Input: part model. Units: mm. Frame: model coordinates. A direction names the side the tool comes from. Give positions to 0.01 mm unless a question says otherwise; leave off trailing zeros. Loops run counter-clockwise (first coordinate to the right, second up) from the corner with the lowest first, then second, coordinate; pieces in that order, holes last. Notation, with made-up numbers: M 0.5,66 L 46.5,66 A6 ccw 46.5,76 Z; hole C 50,76.5 d8. An arc over 180 degrees is marked long. Return JSON: item names as keys, results as strings. Group by question number.
```python
from build123d import *

# Parameters (mm, degrees)
PAD002_DEPTH     = 75
BOX011_W         = 66
BOX011_H         = 16
BOX011_DEPTH     = 0.75
BOX010_W         = 0.75
BOX010_H         = 0.75
BOX010_DEPTH     = 9
ARRAY007_X_COUNT = 2
ARRAY007_X_PITCH = 70.45
ARRAY007_Y_COUNT = 2
ARRAY007_Y_PITCH = 24.45
BOX009_W         = 71.2
BOX009_H         = 25.2
BOX009_DEPTH     = 8.9


with BuildPart() as screen_lateral_hole:
    # Sketch002 → Pad002 (new body)
    with BuildSketch(Plane.YZ):
        Polygon((12.982779, 1.619702), (12.982779, 4.769702), (15.482779, 4.769702), (15.482779, 6.269702), (30.482779, 6.269702), (30.482779, 4.769702), (32.982779, 4.769702), (32.982779, 1.619702), align=None)
    extrude(amount=PAD002_DEPTH)


with BuildPart() as screen_lateral_hole_1:
    # Body002 placement: moved
    add(screen_lateral_hole.part.moved(Location((9, 0, 0))))


with BuildPart() as screen:
    # Box011 → Box011 (new body)
    with BuildSketch(Plane(origin=(9, 15, 9.75), x_dir=(1, 0, 0), z_dir=(0, 0, 1))):
        with Locations((33, 8)):
            Rectangle(BOX011_W, BOX011_H)
    extrude(amount=BOX011_DEPTH)


with BuildPart() as obj1:
    # Box010 → Box010 (new body)
    with BuildSketch(Plane(origin=(6.4, 10.4, 1.6), x_dir=(1, 0, 0), z_dir=(0, 0, 1))):
        with Locations((0.375, 0.375)):
            Rectangle(BOX010_W, BOX010_H)
    extrude(amount=BOX010_DEPTH)

    # Array007 X: obj1_2


with BuildPart() as obj1_1:
    add(obj1.part)
    with Locations(*[(i * ARRAY007_X_PITCH, 0, 0) for i in range(1, ARRAY007_X_COUNT)]):
        add(obj1.part)

    # Array007 Y: obj1_2


with BuildPart() as obj1_2:
    add(obj1_1.part)
    with Locations(*[(0, i * ARRAY007_Y_PITCH, 0) for i in range(1, ARRAY007_Y_COUNT)]):
        add(obj1_1.part)

    # Fusion002004: union Screen Lateral Hole, Screen
    add(screen_lateral_hole_1.part)
    add(screen.part)


with BuildPart() as panel:
    # Box009 → Box009 (new body)
    with BuildSketch(Plane(origin=(6.4, 10.4, 1.6), x_dir=(1, 0, 0), z_dir=(0, 0, 1))):
        with Locations((35.6, 12.6)):
            Rectangle(BOX009_W, BOX009_H)
    extrude(amount=BOX009_DEPTH)

    # Cut001: cut obj1
    add(obj1_2.part, mode=Mode.SUBTRACT)


solid = panel.part
```
Item 1: Section B-B, the plane z = 5.5. Return loops of the section in (x, y).
Item 2: Section A-A, the plane x = 51.5. Return loops of the section in (y, z).
Item 3: First-contact query: pin 1 Ø3.5 at (y, z) = (27, 3.5) entering from +X. Flat tip, straight axial feed; report the tip coordinate or a pass-through.
Item 4: Reachability of faces 4 (the face through (6.4, 23, 6)), 5 (the face through (43, 15.483, 6)) from +Z, -Z, +X, -X, +Y, -Y: full face, straight path, thin tool, end or side. Return the list, or none.
Item 5: Material intervals for line 1 (Y direction, x = 20, z = 2); line 2 (X direction, y = 22, z = 10); line 3 (Y direction, x = 41.5, z = 10), sorted ascending. Write a range as from..to.
Item 6: Pull-direction query (Z, two-part tool) for faces 1 (the face through (43, 14, 4.77)), 2 (the face through (42, 10.4, 6)), 3 (the face through (42, 23, 9.75)); classes: pulls with the +Z half, pulls with the -Z half, needs draft (parallel to the pull), parting line crosses it, or undercut.
Answer below:
{
 "1": {"outline": "M 6.4,11.15 L 7.15,11.15 L 7.15,10.4 L 76.85,10.4 L 76.85,11.15 L 77.6,11.15 L 77.6,15.48 L 9,15.48 L 9,30.48 L 77.6,30.48 L 77.6,34.85 L 76.85,34.85 L 76.85,35.6 L 7.15,35.6 L 7.15,34.85 L 6.4,34.85 Z"},
 "2": {"outline": "M 10.4,1.6 L 35.6,1.6 L 35.6,10.5 L 31,10.5 L 31,9.75 L 15,9.75 L 15,10.5 L 10.4,10.5 Z; hole M 12.98,1.62 L 32.98,1.62 L 32.98,4.77 L 30.48,4.77 L 30.48,6.27 L 15.48,6.27 L 15.48,4.77 L 12.98,4.77 Z"},
 "3": {"pin 1": "x = 9"},
 "4": {"face 4": "+Z, -Z, -X, +Y, -Y", "face 5": "+X"},
 "5": {"line 1": "10.4..12.98, 32.98..35.6", "line 2": "6.4..9, 75..77.6", "line 3": "10.4..15, 31..35.6"},
 "6": {"face 1": "undercut", "face 2": "needs draft", "face 3": "pulls with the +Z half"}
}
